Source: CAD feature listing. Evaluate the final solid. Frame: model axes, mm. Face numbers are marked on the shaded views. A direction names the side the tool comes from. Give positions to 0.01 mm unless a question says otherwise; leave off trailing zeros. Loops run counter-clockwise (first coordinate to the right, second up) from the corner with the lowest first, then second, coordinate; pieces in that order, holes last. Notation, with made-up numbers: (4, -31) -> (49, -31) arc R27 ccw to (49, -1) -> close; hole circle Ø5 at (63, 37). An arc over 180 degrees is marked (long way). Put each result on its own line as item: value.
```python
from build123d import *

# Parameters (mm, degrees)
F0_R     = 12.5
F0_R_2   = 22.5
F1_DEPTH = 10
F2_DEPTH = 15
F3_DEPTH = 45


with BuildPart() as f1:
    # F0 (on Front) → F1 (new body, symmetric)
    with BuildSketch(Plane.XZ):
        with BuildLine():
            ThreePointArc((-97.287398, 125.439875), (-91.913374, 118.536626), (-90, 110))
            ThreePointArc((-90, 110), (-103.24713, 91.174519), (-125.439875, 97.287398))
            Line((-125.439875, 97.287398), (-27.019781, -22.247054))
            ThreePointArc((-27.019781, -22.247054), (-24.748737, 24.748738), (22.247054, 27.019781))
            Line((22.247054, 27.019781), (-97.287398, 125.439875))
        make_face()
        with BuildLine():
            Line((24.700145, 25), (24.494897, 25))
            ThreePointArc((24.494897, 25), (32.267022, 13.558735), (35, 0))
            ThreePointArc((35, 0), (32.267022, -13.558735), (24.494897, -25))
            Line((24.494897, -25), (70, -25))
            Line((70, -25), (70, 25))
            Line((70, 25), (24.700145, 25))
        make_face()
        with BuildLine():
            ThreePointArc((-125.439875, 97.287398), (-103.24713, 91.174519), (-90, 110))
            ThreePointArc((-90, 110), (-91.913374, 118.536626), (-97.287398, 125.439875))
            ThreePointArc((-97.287398, 125.439875), (-124.142136, 124.142136), (-125.439875, 97.287398))
        make_face()
        with Locations((-110, 110)):
            Circle(F0_R, mode=Mode.SUBTRACT)
        with BuildLine():
            ThreePointArc((24.494897, 25), (23.392785, 26.034162), (22.247054, 27.019781))
            ThreePointArc((22.247054, 27.019781), (-24.748737, 24.748738), (-27.019781, -22.247054))
            ThreePointArc((-27.019781, -22.247054), (-1.867736, -34.95013), (24.494897, -25))
            ThreePointArc((24.494897, -25), (32.267022, -13.558735), (35, 0))
            ThreePointArc((35, 0), (32.267022, 13.558735), (24.494897, 25))
        make_face()
        Circle(F0_R_2, mode=Mode.SUBTRACT)
        with BuildLine():
            ThreePointArc((110, 25), (90, 45), (70, 25))
            Line((70, 25), (70, -25))
            ThreePointArc((70, -25), (90, -45), (110, -25))
            Line((110, -25), (110, 25))
        make_face()
        with BuildLine():
            ThreePointArc((80, 25), (90, 35), (100, 25))
            Line((100, 25), (100, -25))
            ThreePointArc((100, -25), (90, -35), (80, -25))
            Line((80, -25), (80, 25))
        make_face(mode=Mode.SUBTRACT)
    extrude(amount=F1_DEPTH, both=True)

    # F0 (on Front) → F2 (join, symmetric)
    with BuildSketch(Plane.XZ):
        with BuildLine():
            ThreePointArc((110, 25), (90, 45), (70, 25))
            Line((70, 25), (70, -25))
            ThreePointArc((70, -25), (90, -45), (110, -25))
            Line((110, -25), (110, 25))
        make_face()
        with BuildLine():
            ThreePointArc((80, 25), (90, 35), (100, 25))
            Line((100, 25), (100, -25))
            ThreePointArc((100, -25), (90, -35), (80, -25))
            Line((80, -25), (80, 25))
        make_face(mode=Mode.SUBTRACT)
        with BuildLine():
            ThreePointArc((-125.439875, 97.287398), (-103.24713, 91.174519), (-90, 110))
            ThreePointArc((-90, 110), (-91.913374, 118.536626), (-97.287398, 125.439875))
            ThreePointArc((-97.287398, 125.439875), (-124.142136, 124.142136), (-125.439875, 97.287398))
        make_face()
        with Locations((-110, 110)):
            Circle(F0_R, mode=Mode.SUBTRACT)
    extrude(amount=F2_DEPTH, both=True)

    # F0 (on Front) → F3 (join, symmetric)
    with BuildSketch(Plane.XZ):
        with BuildLine():
            ThreePointArc((24.494897, 25), (23.392785, 26.034162), (22.247054, 27.019781))
            ThreePointArc((22.247054, 27.019781), (-24.748737, 24.748738), (-27.019781, -22.247054))
            ThreePointArc((-27.019781, -22.247054), (-1.867736, -34.95013), (24.494897, -25))
            ThreePointArc((24.494897, -25), (32.267022, -13.558735), (35, 0))
            ThreePointArc((35, 0), (32.267022, 13.558735), (24.494897, 25))
        make_face()
        Circle(F0_R_2, mode=Mode.SUBTRACT)
    extrude(amount=F3_DEPTH, both=True)


solid = f1.part
```
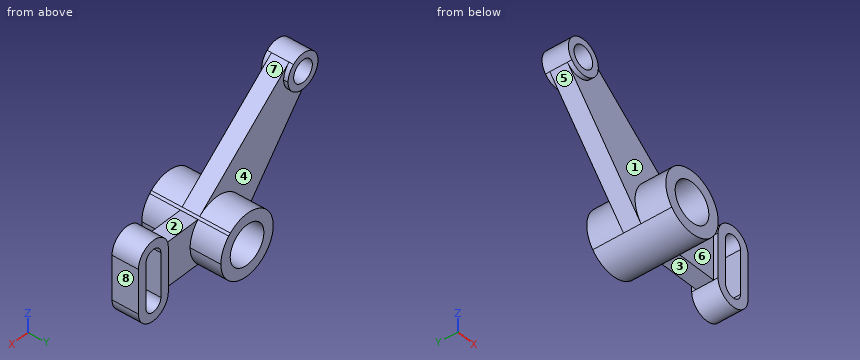
(1) Draft query along X for the marked faces 5, 6, 7 and 8. Return one class per face: released by +X, released by -X, zero draft, split by the parting line, or undercut.
Calculated:
face 5: released by -X
face 6: undercut
face 7: undercut
face 8: released by +X
(2) First-contact query: P1, Ø12, axis at y = -25, z = -26, coming from the +X side; P2, Ø16, axis at x = 44.5, y = -3, coming from the +Z side; P3, Ø4, axis at x = -104.5, y = 10.5, coming from the +Z side. Flat tips, straight axial feed; report the tip coordinate or a pass-through.
Calculated:
P1: stops at x = 28.72
P2: stops at z = 25
P3: stops at z = 129.69
(3) Section D-D on z = -15. Return loops of the section in (x, y), then the cut area to 3 significant figures.
Calculated:
outline: (-32.99, -10) -> (-31.62, -10) -> (-31.62, -45) -> (-16.77, -45) -> (-16.77, 45) -> (-31.62, 45) -> (-31.62, 10) -> (-32.99, 10) -> close; (16.77, -45) -> (31.62, -45) -> (31.62, -10) -> (70, -10) -> (70, -15) -> (80, -15) -> (80, 15) -> (70, 15) -> (70, 10) -> (31.62, 10) -> (31.62, 45) -> (16.77, 45) -> close; (100, -15) -> (110, -15) -> (110, 15) -> (100, 15) -> close
area: 4,070 mm²
(4) Line query: probe 1 along Z at (x, y) = (0, -23); probe 2 along Z at (x, y) = (-116, -0.5); probe 3 along Y at (x, z) = (73.5, -30). Output: solid intervals per line, ascending. Write a range as from..to.
Calculated:
probe 1: z = -35..-22.5, 22.5..35
probe 2: z = 85.82..99.03, 120.97..129.08
probe 3: y = -15..15
(5) Reachability of the marked faces 1, 2, 3 and 4 from +Z, -Z, +X, -X, +Y, -Y: full face, straight path, thin tool, end or side. Return the list, or none.
Calculated:
face 1: -Y
face 2: +Z, +Y, -Y
face 3: -Z, +Y, -Y
face 4: +Y
(6) Section A-A on x = 90. Return loops of the section in (y, z).
Calculated:
outline: (-15, -45) -> (15, -45) -> (15, -35) -> (-15, -35) -> close; (-15, 35) -> (15, 35) -> (15, 45) -> (-15, 45) -> close
(7) Section B-B on z = 105. Return loops of the section in (x, y), then the cut area to 3 significant figures.
Calculated:
outline: (-129.36, -15) -> (-121.46, -15) -> (-121.46, 15) -> (-129.36, 15) -> close; (-98.54, -15) -> (-90.64, -15) -> (-90.64, -10) -> (-72.46, -10) -> (-72.46, 10) -> (-90.64, 10) -> (-90.64, 15) -> (-98.54, 15) -> close
area: 838 mm²
(8) Section C-C on y = -32.5. Return loops of the section in (x, z), then the cut area to 3 significant figures.
Calculated:
outline: (-27.02, -22.25) arc R35 ccw to (24.49, -25) arc R35 ccw to (35, 0) arc R35 ccw to (24.49, 25) arc R35 ccw to (22.25, 27.02) arc R35 ccw to start; hole circle Ø45 at (0, 0)
area: 2,260 mm²
